Verification items for this drawing (mm, ordinates from the low corner). Round coordinates to 2 decimals unless told otherwise and drop trailing zeros. Loops run counter-clockwise (first coordinate to the right, second up) from the corner with the lowest first, then second, coordinate; pieces in that order, holes last. Notation, with made-up numbers: (3, 79.5) -> (41, 79.5) arc R19 ccw to (41, 109.5) -> close; hole circle Ø8 at (34, 56.5). An arc over 180 degrees is marked (long way). Use a Markdown table: item, result. Add a question column.
Q1. Gauge pin test, flat ends, axial feed: P1, Ø2, axis at x = 19.5, z = 1, coming from the +Y side; P2, Ø5, axis at x = 15, y = 30, coming from the +Z side. Record the tip position at first contact, or that the pin passes through.
Q2. Material ranges on L1, parallel to Y at x = 15, z = 2 (3 decimals); L2, parallel to X at y = 38, z = 3.75; L3, parallel to X at y = 35, z = 1.5, recorded low to high.
Q3. Sectioned sample at B-B, the plane z = 1.75. Enter the section's corners in (x, y) (3 decimals).
Q4. Sectioned sample at D-D, the plane y = 38.5. Enter the section's corners in (x, z).
Q5. Sectioned sample at A-A, the plane x = 15. Enter the section's corners in (y, z) (3 decimals).
Q6. Sectioned sample at C-C, the plane y = 29. Enter the section's corners in (x, z).
Q7. Release check for a two-part mould opening along X. For the marked faces 1, 2, 3 and 4 record: released by +X, released by -X, zero draft, split by the parting line, or undercut.
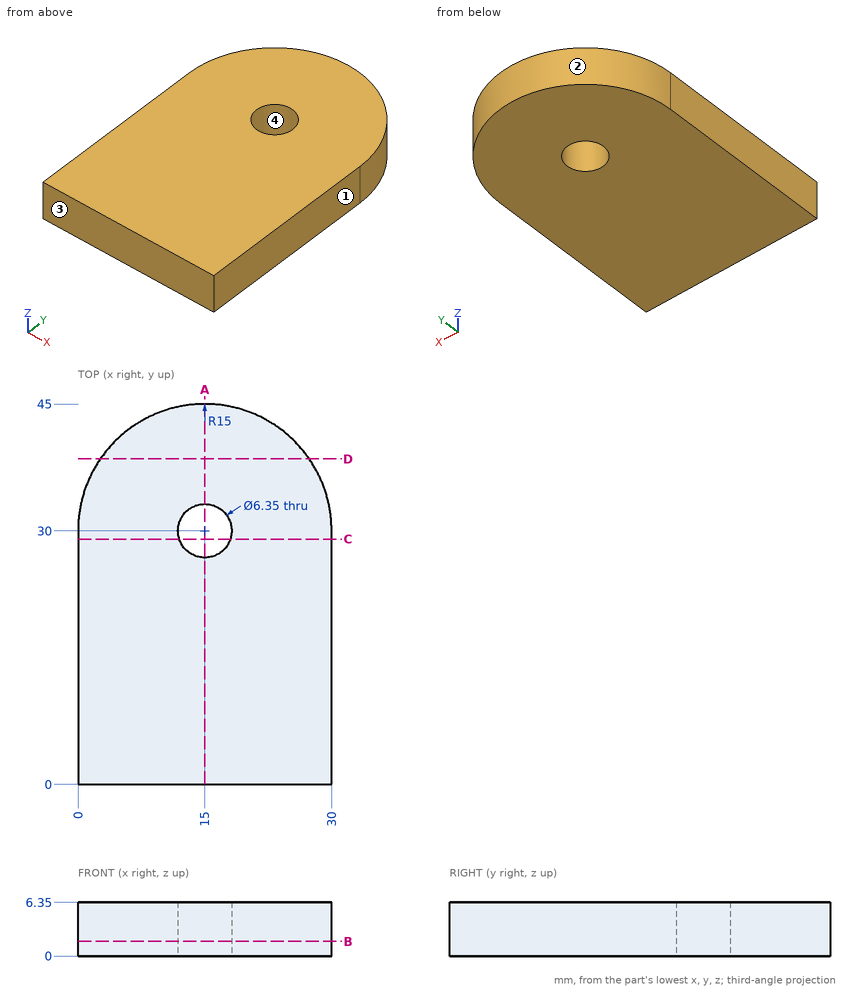
Values:
| question | item | result |
|---|---|---|
| 1 | P1 | y = 44.59 |
| 1 | P2 | through |
| 2 | L1 | 0 to 26.825, 33.175 to 45 |
| 2 | L2 | 2.31 to 27.69 |
| 2 | L3 | 0.86 to 29.14 |
| 3 | outline | (0, 0) -> (30, 0) -> (30, 30) arc R15 ccw to (0, 30) -> close; hole circle Ø6.35 at (15, 30) |
| 4 | outline | (2.64, 0) -> (27.36, 0) -> (27.36, 6.35) -> (2.64, 6.35) -> close |
| 5 | outline | (0, 0) -> (26.825, 0) -> (26.825, 6.35) -> (0, 6.35) -> close; (33.175, 0) -> (45, 0) -> (45, 6.35) -> (33.175, 6.35) -> close |
| 6 | outline | (0, 0) -> (11.99, 0) -> (11.99, 6.35) -> (0, 6.35) -> close; (18.01, 0) -> (30, 0) -> (30, 6.35) -> (18.01, 6.35) -> close |
| 7 | face 1 | released by +X |
| 7 | face 2 | split by the parting line |
| 7 | face 3 | zero draft |
| 7 | face 4 | undercut |
